The model under review builds one solid part; all positions refer to its coordinate system, in mm. A direction names the side the tool comes from. Give positions to 0.01 mm unless a question says otherwise; leave off trailing zeros. Order: outer loops, then holes, each group sorted by start corner. A loop starts at its lowest first (then second) coordinate and runs counter-clockwise, first axis right, second up.
```python
from build123d import *

# Parameters (mm, degrees)
SKETCH1_R           = 10
SKETCH1_R_2         = 2.65
BOSS_EXTRUDE1_DEPTH = 1
SKETCH2_R           = 10
SKETCH4_R           = 20
SKETCH3_R           = 30
SKETCH5_R           = 11.5
SKETCH5_R_2         = 10
BOSS_EXTRUDE2_DEPTH = 1
SKETCH10_R          = 51.016643615
CUT_EXTRUDE2_DEPTH  = 70
FILLET1_R           = 1
SKETCH12_R          = 1
SKETCH12_R_2        = 1.5
CUT_EXTRUDE4_DEPTH  = 10


with BuildPart() as part:
    # Sketch1 → Boss-Extrude1 (new body)
    with BuildSketch(Plane.XY):
        Circle(SKETCH1_R)
        with Locations((0, 6)):
            Circle(SKETCH1_R_2, mode=Mode.SUBTRACT)
        with Locations((5.706339098, 1.854101966)):
            Circle(SKETCH1_R_2, mode=Mode.SUBTRACT)
        with Locations((3.526711514, -4.854101966)):
            Circle(SKETCH1_R_2, mode=Mode.SUBTRACT)
        with Locations((-3.526711514, -4.854101966)):
            Circle(SKETCH1_R_2, mode=Mode.SUBTRACT)
        with Locations((-5.706339098, 1.854101966)):
            Circle(SKETCH1_R_2, mode=Mode.SUBTRACT)
    extrude(amount=BOSS_EXTRUDE1_DEPTH)



with BuildPart() as body_2:
    # Sketch2 → Loft-Thin1 section 0
    with BuildSketch(Plane.XY.offset(1)):
        Circle(SKETCH2_R)
    # Sketch4 → Loft-Thin1 section 1
    with BuildSketch(Plane.XY.offset(15)):
        Circle(SKETCH4_R)
    # Sketch3 → Loft-Thin1 section 2
    with BuildSketch(Plane.XY.offset(45)):
        Circle(SKETCH3_R)
    loft()


with BuildPart() as part_1:
    add(part.part)

    add(body_2.part)  # Boss-Extrude2 merges body 2
    # Sketch5 → Boss-Extrude2 (add)
    with BuildSketch(Plane(origin=(0, 0, 0), x_dir=(-1, 0, 0), z_dir=(0, 0, -1))):
        Circle(SKETCH5_R)
        Circle(SKETCH5_R_2, mode=Mode.SUBTRACT)
    extrude(amount=-BOSS_EXTRUDE2_DEPTH)

    # Sketch10 → Cut-Extrude2 (cut)
    with BuildSketch(Plane.XY):
        Circle(SKETCH10_R)
    extrude(amount=CUT_EXTRUDE2_DEPTH, mode=Mode.SUBTRACT)


with BuildPart() as body_2_2:
    # Sketch8 → Revolve1 (revolve)
    with BuildSketch(Plane(origin=(0, 0, 0), x_dir=(0, 0, -1), z_dir=(1, 0, 0))):
        Polygon((0, 18.5), (18.5, 18.5), (18.5, 0), (20, 0), (20, 20), (0, 20), align=None)
    revolve(axis=Axis((0, 0, -20), (0, 0, 1)))

    # Fillet1
    fillet1_edges = [body_2_2.edges().sort_by_distance(p)[0] for p in [
        (0, -18.5, -18.5),
    ]]
    fillet(fillet1_edges, radius=FILLET1_R)

    # Sketch12 → Cut-Extrude4 (cut)
    with BuildSketch(Plane.XY.offset(-18.5)):
        with Locations((0, 5)):
            Circle(SKETCH12_R)
        with Locations((0, -5)):
            Circle(SKETCH12_R)
        Circle(SKETCH12_R_2)
    extrude(amount=-CUT_EXTRUDE4_DEPTH, mode=Mode.SUBTRACT)


solid = body_2_2.part
```
Item 1: Clearance check with flat-ended pins moving along their axes: pin 1 Ø2 at (x, y) = (0, 1) entering from -Z; pin 2 Ø12 at (y, z) = (0.5, -11) entering from +X; pin 3 Ø2 at (x, z) = (-10.5, -5) entering from -Y; pin 4 Ø5 at (x, y) = (0, 0) entering from +Z. State where each tip first meets the part, or that it passes through.
Values found:
pin 1: stops at z = -20
pin 2: stops at x = 20
pin 3: stops at y = -17.6
pin 4: stops at z = -18.5
Item 2: Take a section at B-B (z = -12.25). Give the boundary of the cut face in (x, y), and give its area (3 significant figures).
Values found:
outline: circle Ø40 at (0, 0); hole circle Ø37 at (0, 0)
area: 181 mm2
Item 3: For line 1 (Y direction, x = 0, z = -19.7); line 2 (Y direction, x = 0.5, z = -2); line 3 (X direction, y = 0, z = -11.25), list the stretches that pass through material, from the lowest coordinate up.
Values found:
line 1: y = -20 to -6, -4 to -1.5, 1.5 to 4, 6 to 20
line 2: y = -19.99 to -18.49, 18.49 to 19.99
line 3: x = -20 to -18.5, 18.5 to 20
Item 4: For faces 1 (the cylindrical face through (18.06, -4.01, -8.87)), 2 (the cylindrical face through (-1.5, 0.07, -19.24)), list the 3-axis set-ups (+Z, -Z, +X, -X, +Y, -Y) from which the entire face can be reached by the end or side of a thin tool; tool diameter is ignored.
Values found:
face 1: +Z
face 2: +Z, -Z
Item 5: Take a section at A-A (x = 0). Give the boundary of the cut face in (y, z), and give its area (3 significant figures).
Values found:
outline: (-20, -20) - (-6, -20) - (-6, -18.5) - (-17.5, -18.5) arc R1 cw to (-18.5, -17.5) - (-18.5, 0) - (-20, 0) - close; (-4, -20) - (-1.5, -20) - (-1.5, -18.5) - (-4, -18.5) - close; (1.5, -20) - (4, -20) - (4, -18.5) - (1.5, -18.5) - close; (6, -20) - (20, -20) - (20, 0) - (18.5, 0) - (18.5, -17.5) arc R1 cw to (17.5, -18.5) - (6, -18.5) - close
area: 105 mm2
Item 6: Draft analysis for pull direction Y (two halves, no side actions). For faces 3 (the cylindrical face through (19.524, -4.336, -9.86)), 4 (the cylindrical face through (0, -4, -19)), 5 (the flat face through (18, 6, 0)), state which applies: released by +Y, released by -Y, zero draft, split by the parting line, or undercut.
Values found:
face 3: split by the parting line
face 4: undercut
face 5: zero draft
